Source: CAD feature listing. Evaluate the final solid. Frame: model axes, mm. A direction names the side the tool comes from. Give positions to 0.01 mm unless a question says otherwise; leave off trailing zeros. Order: outer loops, then holes, each group sorted by start corner. A loop starts at its lowest first (then second) coordinate and runs counter-clockwise, first axis right, second up.
from build123d import *

# Parameters (mm, degrees)
F0_W     = 60
F0_H     = 40
F1_DEPTH = 10
F5_DEPTH = 20


# Not quite as in the source:
# - a feature of the source that left no trace in its solid (it failed there, or was rolled back) is left out


with BuildPart() as f1:
    # F0 (on Top) → F1 (new body)
    with BuildSketch(Plane.XY):
        with Locations((30, 20)):
            Rectangle(F0_W, F0_H)
    extrude(amount=F1_DEPTH)

    # F2 (on Front) → F5 (join)
    with BuildSketch(Plane.XZ):
        with BuildLine():
            Line((49.8285376106, 20), (40, 20))
            ThreePointArc((40, 20), (20, 40), (0, 20))
            Line((0, 20), (0, 10.3115513921))
            Line((0, 10.3115513921), (59.8550215364, 9.9916663021))
            Line((59.8550215364, 9.9916663021), (59.8027205061, 10.7181055402))
            ThreePointArc((59.8027205061, 10.7181055402), (56.6409874121, 17.3205551498), (49.8285376106, 20))
        make_face()
    extrude(amount=-F5_DEPTH)


solid = f1.part
1) First-contact query: pin 1 Ø9 at (x, z) = (37, 28) entering from +Y; pin 2 Ø11 at (x, y) = (44, 9.5) entering from +Z; pin 3 Ø8 at (y, z) = (12.5, 33.5) entering from -X. Flat tips, straight axial feed; report the tip coordinate or a pass-through.
Checks:
pin 1: stops at y = 20
pin 2: stops at z = 27.6
pin 3: stops at x = 2.4
2) Pull-direction query (Z, two-part tool) for faces 3 (the face through (30, 40, 5)), 4 (the face through (30, 20, 10)), 5 (the face through (45, 10, 20)); classes: +Z half, -Z half, draft (parallel to the pull), parting line (faces both ways), or undercut.
Checks:
face 3: draft
face 4: undercut
face 5: +Z half
3) Section query A-A on x = 8.5. Output: boundary loops of the cut face in (y, z).
Checks:
outline: (0, 0) - (40, 0) - (40, 10) - (0, 10) - close; (0, 10.27) - (20, 10.27) - (20, 36.36) - (0, 36.36) - close
4) Reachability of faces 1 (the face through (23, 20, 22)), 2 (the face through (56.717, 9.86, 17.249)) from +Z, -Z, +X, -X, +Y, -Y: full face, straight path, thin tool, end or side. Return the list, or none.
Checks:
face 1: +Z, +X, -X, +Y
face 2: +Z, +X, +Y, -Y
5) Section query B-B on y = 9.5. Output: boundary loops of the cut face in (x, z), and give its area (3 significant figures).
Checks:
outline: (0, 0) - (60, 0) - (60, 10) - (59.85, 10) - (59.8, 10.72) arc R10 ccw to (49.83, 20) - (40, 20) arc R20 ccw to (0, 20) - (0, 10.31) - (58.3, 10) - (0, 10) - close
area: 1,800 mm2
6) Section query C-C on x = 56.5. Output: boundary loops of the cut face in (y, z).
Checks:
outline: (0, 0) - (40, 0) - (40, 10) - (0, 10) - close; (0, 10.01) - (20, 10.01) - (20, 17.45) - (0, 17.45) - close
7) Ray query, L1, parallel to Z at x = 29, y = 4; L2, parallel to Y at x = 41, z = 18.5; L3, parallel to Z at x = 13, y = 3 (3 decimals). Return the intervals inside material, ascending.
Checks:
L1: z = 0 to 10, 10.16 to 37.86
L2: y = 0 to 20
L3: z = 0 to 10, 10.242 to 38.735
8) Section query D-D on z = 29.5. Output: boundary loops of the cut face in (x, y), and give its area (3 significant figures).
Checks:
outline: (2.4, 0) - (37.6, 0) - (37.6, 20) - (2.4, 20) - close
area: 704 mm2
